```python
from build123d import *

# Parameters (mm, degrees)
EXTRUDE_8_DEPTH        = 4
EXTRUDE_8_DEPTH_BACK   = 4
EXTRUDE_9_DEPTH        = 5
EXTRUDE_9_DEPTH_BACK   = 5
EXTRUDE_10_DEPTH       = 2
EXTRUDE_10_DEPTH_BACK  = 2
EXTRUDE_11_DEPTH       = 3
EXTRUDE_11_DEPTH_BACK  = 3
EXTRUDE_12_DEPTH       = 3
EXTRUDE_12_DEPTH_BACK  = 3
EXTRUDE_13_DEPTH       = 6
EXTRUDE_13_DEPTH_BACK  = 6
HOLE_WIZARD_M6_2_D     = 5
HOLE_WIZARD_M6_2_DEPTH = 15
HOLE_WIZARD_M6_2_TIP   = 1.502151548


with BuildPart() as part:
    # Sketch 1 → Extrude 8 (new, two sides: drawn at the far end of the back side and taken through both)
    with BuildSketch(Plane.XY.offset(-EXTRUDE_8_DEPTH_BACK)):
        with BuildLine():
            Line((69.5, 0), (0, 0))
            Line((0, 0), (0, -14))
            Line((0, -14), (3.5, -14))
            Line((3.5, -14), (65.5, -22.713531752))
            Line((65.5, -22.713531752), (69.5, -22.713531752))
            Line((69.5, -22.713531752), (69.5, -18.936822587))
            ThreePointArc((69.5, -18.936822587), (69.221207402, -18.208623367), (69, -17.460915736))
            Line((69, -17.460915736), (69, -13))
            ThreePointArc((69, -13), (69.127016654, -12), (69.5, -11.063508327))
            Line((69.5, -11.063508327), (69.5, 0))
        make_face()
        with BuildLine():
            Line((65.5, -22.713531752), (3.5, -14))
            Line((3.5, -14), (3.5, -54))
            Line((3.5, -54), (14, -55.475678764))
            Line((14, -55.475678764), (14, -32.5))
            ThreePointArc((14, -32.5), (15.171572875, -29.671572875), (18, -28.5))
            Line((18, -28.5), (24, -28.5))
            ThreePointArc((24, -28.5), (26.828427125, -29.671572875), (28, -32.5))
            Line((28, -32.5), (28, -57.44325045))
            Line((28, -57.44325045), (42, -59.410822136))
            Line((42, -59.410822136), (42, -32.5))
            ThreePointArc((42, -32.5), (43.171572875, -29.671572875), (46, -28.5))
            Line((46, -28.5), (52, -28.5))
            ThreePointArc((52, -28.5), (54.828427125, -29.671572875), (56, -32.5))
            Line((56, -32.5), (56, -61.378393822))
            Line((56, -61.378393822), (65.5, -62.713531752))
            Line((65.5, -62.713531752), (65.5, -28.095746335))
            ThreePointArc((65.5, -28.095746335), (67.655069896, -24.546629134), (71.798116456, -24.821809752))
            ThreePointArc((71.798116456, -24.821809752), (70.580276552, -23.842645827), (69.5, -22.713531752))
            Line((69.5, -22.713531752), (65.5, -22.713531752))
        make_face()
    extrude(amount=EXTRUDE_8_DEPTH + EXTRUDE_8_DEPTH_BACK)

    # Sketch 1_10 → Extrude 9 (add, two sides: drawn at the far end of the back side and taken through both)
    with BuildSketch(Plane.XY.offset(-EXTRUDE_9_DEPTH_BACK)):
        with BuildLine():
            Line((130, 0), (69.5, 0))
            Line((69.5, 0), (69.5, -11.063508327))
            ThreePointArc((69.5, -11.063508327), (70.968493994, -9.554280431), (73, -9))
            Line((73, -9), (77.08693273, -9))
            Line((77.08693273, -9), (83.5, -9))
            ThreePointArc((83.5, -9), (86.328427125, -10.171572875), (87.5, -13))
            Line((87.5, -13), (87.5, -18.58993247))
            ThreePointArc((87.5, -18.58993247), (87.296056581, -19.850866423), (86.705022784, -20.983220784))
            ThreePointArc((86.705022784, -20.983220784), (80.974921845, -24.736035873), (74.173945542, -23.920929013))
            ThreePointArc((74.173945542, -23.920929013), (71.398076595, -21.840459472), (69.5, -18.936822587))
            Line((69.5, -18.936822587), (69.5, -22.713531752))
            ThreePointArc((69.5, -22.713531752), (70.580276552, -23.842645827), (71.798116456, -24.821809752))
            ThreePointArc((71.798116456, -24.821809752), (77.179945202, -26.904296761), (82.91155309, -26.233846298))
            ThreePointArc((82.91155309, -26.233846298), (85.926197724, -26.316026977), (88.02665093, -28.480035357))
            Line((88.02665093, -28.480035357), (90.262355313, -34.013597882))
            Line((90.262355313, -34.013597882), (95.364949439, -46.642961524))
            Line((95.364949439, -46.642961524), (100.356245485, -58.996852747))
            ThreePointArc((100.356245485, -58.996852747), (103.300173094, -62.63230058), (107.773716321, -64))
            Line((107.773716321, -64), (125.831836464, -64))
            ThreePointArc((125.831836464, -64), (132.895417207, -59.755772502), (132.464137044, -51.526456772))
            Line((132.464137044, -51.526456772), (112.86769942, -22.473543228))
            ThreePointArc((112.86769942, -22.473543228), (111.857848283, -15.634092747), (116.555476326, -10.561600956))
            ThreePointArc((116.555476326, -10.561600956), (124.046039774, -6.258819743), (130, 0))
        make_face()
    extrude(amount=EXTRUDE_9_DEPTH + EXTRUDE_9_DEPTH_BACK)

    # Sketch 1_11 → Extrude 10 (add, two sides: drawn at the far end of the back side and taken through both)
    with BuildSketch(Plane.XY.offset(-EXTRUDE_10_DEPTH_BACK)):
        with BuildLine():
            ThreePointArc((79.837012191, -21.417403525), (77.598679354, -24.011007569), (74.173945542, -23.920929013))
            ThreePointArc((74.173945542, -23.920929013), (80.974921845, -24.736035873), (86.705022784, -20.983220784))
            ThreePointArc((86.705022784, -20.983220784), (87.296056581, -19.850866423), (87.5, -18.58993247))
            Line((87.5, -18.58993247), (87.5, -13))
            ThreePointArc((87.5, -13), (86.328427125, -10.171572875), (83.5, -9))
            Line((83.5, -9), (77.08693273, -9))
            ThreePointArc((77.08693273, -9), (79.956123916, -10.212933095), (81.08524663, -13.116129032))
            ThreePointArc((81.08524663, -13.116129032), (80.710908742, -17.304324748), (79.837012191, -21.417403525))
        make_face()
    extrude(amount=EXTRUDE_10_DEPTH + EXTRUDE_10_DEPTH_BACK)

    # Sketch 1_12 → Extrude 11 (add, two sides: drawn at the far end of the back side and taken through both)
    with BuildSketch(Plane.XY.offset(-EXTRUDE_11_DEPTH_BACK)):
        with BuildLine():
            Line((95.364949439, -46.642961524), (90.262355313, -34.013597882))
            ThreePointArc((90.262355313, -34.013597882), (90.537164852, -35.874473659), (89.931018667, -37.655194228))
            ThreePointArc((89.931018667, -37.655194228), (89.568508885, -41.63940278), (92.596940419, -44.25358211))
            ThreePointArc((92.596940419, -44.25358211), (94.269957944, -45.113460767), (95.364949439, -46.642961524))
        make_face()
    extrude(amount=EXTRUDE_11_DEPTH + EXTRUDE_11_DEPTH_BACK)

    # Sketch 1_13 → Extrude 12 (add, two sides: drawn at the far end of the back side and taken through both)
    with BuildSketch(Plane.XY.offset(-EXTRUDE_12_DEPTH_BACK)):
        with BuildLine():
            Line((14, -32.5), (14, -55.475678764))
            Line((14, -55.475678764), (28, -57.44325045))
            Line((28, -57.44325045), (28, -32.5))
            ThreePointArc((28, -32.5), (26.828427125, -29.671572875), (24, -28.5))
            Line((24, -28.5), (18, -28.5))
            ThreePointArc((18, -28.5), (15.171572875, -29.671572875), (14, -32.5))
        make_face()
        with BuildLine():
            Line((42, -32.5), (42, -59.410822136))
            Line((42, -59.410822136), (56, -61.378393822))
            Line((56, -61.378393822), (56, -32.5))
            ThreePointArc((56, -32.5), (54.828427125, -29.671572875), (52, -28.5))
            Line((52, -28.5), (46, -28.5))
            ThreePointArc((46, -28.5), (43.171572875, -29.671572875), (42, -32.5))
        make_face()
    extrude(amount=EXTRUDE_12_DEPTH + EXTRUDE_12_DEPTH_BACK)

    # Sketch 13 → Extrude 13 (add, two sides: drawn at the far end of the back side and taken through both)
    with BuildSketch(Plane.XY.offset(-EXTRUDE_13_DEPTH_BACK)):
        Polygon((69.5, 0), (69.5, -22.713531752), (3.5, -14), (0, -14), (0, 0), align=None)
    extrude(amount=EXTRUDE_13_DEPTH + EXTRUDE_13_DEPTH_BACK)

    # Hole Wizard M6 _2
    with Locations(Plane(origin=(0, 0, 0), x_dir=(1, 0, 0), z_dir=(0, 1, 0))):
        with Locations((20, 0), (108, 0)):
            Hole(HOLE_WIZARD_M6_2_D / 2, depth=HOLE_WIZARD_M6_2_DEPTH)
            with Locations((0, 0, -(HOLE_WIZARD_M6_2_DEPTH + HOLE_WIZARD_M6_2_TIP / 2))):  # 118° drill point
                Cone(0, HOLE_WIZARD_M6_2_D / 2, HOLE_WIZARD_M6_2_TIP, mode=Mode.SUBTRACT)


solid = part.part
```
The model under review builds one solid part; all positions refer to its coordinate system, in mm. A direction names the side the tool comes from. Coordinates: 2 decimals unless noted, no trailing zeros. Write each loop counter-clockwise with the first axis right and the second up, starting at its lowest first coordinate (ties: lowest second). Pieces come first, ordered by that corner, then holes.
1) Clearance check with flat-ended pins moving along their axes: pin 1 Ø3 at (x, y) = (52.5, -22.5) entering from +Z; pin 2 Ø0.8 at (y, z) = (-40, -3.5) entering from +X; pin 3 Ø1.1 at (x, z) = (50, -3.5) entering from -Y. State where each tip first meets the part, or that it passes through.
2) The part is to be moulded in two halves that separate along X. For faces 1 (the face through (15.141, -29.703, -3.507)), 2 (the face through (35, -9, 6)), 3 (the face through (132.84, -59.86, -0.07)), say which applies: pulls with the +X half, pulls with the -X half, needs draft (parallel to the pull), parting line crosses it, or undercut.
3) We need section A-A on y = -50. State the section outline as (x, z) points.
4) To check wall thickness, follow probe 1 along Z at (x, y) = (20, -6.75); probe 2 along Z at (x, y) = (108, -10.5); probe 3 along Y at (x, z) = (120, 3.5). State the ranges of each line that lie inside material, in increasing order.
5) Machinability: for faces 4 (the face through (30, -33, 4)), 5 (the face through (86.297, -10.141, -3.521)), 6 (the face through (2, -14, 0)), 7 (the face through (54.797, -29.641, -3.507)), which of the approach directions +Z, -Z, +X, -X, +Y, -Y give a long, thin tool a straight path to every point of the face, cutting with its end or side? Answer none if there is none.
Answer list:
1. pin 1: stops at z = 4
1. pin 2: stops at x = 124.96
1. pin 3: stops at y = -60.57
2. face 1: undercut
2. face 2: needs draft
2. face 3: pulls with the +X half
3. outline: (3.5, -4) - (14, -4) - (14, -3) - (28, -3) - (28, -4) - (42, -4) - (42, -3) - (56, -3) - (56, -4) - (65.5, -4) - (65.5, 4) - (56, 4) - (56, 3) - (42, 3) - (42, 4) - (28, 4) - (28, 3) - (14, 3) - (14, 4) - (3.5, 4) - close; (96.72, -5) - (131.43, -5) - (131.43, 5) - (96.72, 5) - close
4. probe 1: z = -6 to -2.5, 2.5 to 6
4. probe 2: z = -5 to -2.5, 2.5 to 5
4. probe 3: y = -64 to -33.05, -8.94 to 0
5. face 4: +Z, -X, -Y
5. face 5: -Z
5. face 6: +Z, -Z, -X, -Y
5. face 7: -Z, -Y
